Input: part model. Units: mm. Frame: model coordinates. A direction names the side the tool comes from. Coordinates: 2 decimals unless noted, no trailing zeros. Loops run counter-clockwise (first coordinate to the right, second up) from the corner with the lowest first, then second, coordinate; pieces in that order, holes last.
(1) Section C-C, the plane x = 3. Return loops of the section in (y, z), then the cut area to 3 significant figures.
(2) Contact query for flat-ended pins moving along their axis: P1, Ø3, axis at y = 16.5, z = 2, coming from the -X side; P2, Ø1.5, axis at y = -15, z = 4.5, coming from the -X side; P3, Ø1.1, axis at y = -20.5, z = 5.5, coming from the +X side. Output: stop coordinate, or through.
(3) Set-up query: faces 5 (the face through (-16.17, 16.26, 2.44)), 6 (the face through (-19.6, -10, 5.4)), 7 (the face through (10, -19.8, 5.4)), 8 (the face through (-10, 19.7, 5.4)), 9 (the face through (17.2, 12.4, 5.4)). Return all of +Z, -Z, +X, -X, +Y, -Y with unobstructed straight access to the full face (end or side cutting, diameter ignored); none if empty.
(4) Mould query, pull axis Y, two halves, no side actions, for faces 1 (the face through (17.2, -12.6, 5.4)), 2 (the face through (0, 0, 0.9)), 3 (the face through (-12.4, 16.86, 5.4)), 4 (the face through (12.6, -17.14, 5.4)). Classes: released by +Y, released by -Y, zero draft, split by the parting line, or undercut.
(5) Section B-B, the plane z = 3. Return loops of the section in (x, y).
(6) Section D-D, the plane x = -13.5. Return loops of the section in (y, z), then the cut area to 3 significant figures.
(7) Line query: L1, parallel to Y at x = 0, z = 4.4; L2, parallel to X at y = -0.5, z = 4.2. Output: solid intervals per line, ascending.
(8) Section A-A, the plane y = 0. Return loops of the section in (x, z).
Autodesk Inventor part; units mm, degrees
ref_plane "YZ Plane" through (0, 0, 0) normal (1, 0, 0) x (0, 1, 0)
ref_plane "XZ Plane" through (0, 0, 0) normal (0, 1, 0) x (-1, 0, 0)
ref_plane "XY Plane" through (0, 0, 0) normal (0, 0, 1) x (1, 0, 0)
ref_plane "Work Plane1" through (15.4052, 15.0652, 4.9) normal (0, 0, 1) x (0, 1, 0)
sketch "Sketch1" plane through (15.4052, 15.0652, 4.9) normal (0, 0, 1) x (0, 1, 0)
  circle A0 centre (5.7948, 15.4052) radius 2.5
  circle A1 centre (-15.6052, -5.7948) radius 2.5
  line L0 (-20.0856, 39.0762) -> (-20.0856, 40.2052)
  line L1 (-20.0856, 40.2052) -> (-38.2052, 40.2052)
  arc A2 (-38.2052, 40.2052) -> (-40.2052, 38.2052) centre (-38.2052, 38.2052) ccw
  line L2 (-40.2052, 20.2953) -> (-40.2052, 38.2052)
  line L3 (-40.2052, 20.2953) -> (-39.0783, 20.2953)
  arc A3 (-39.0783, 20.2953) -> (-38.6768, 20.6232) centre (-39.0783, 20.7051) ccw
  arc A4 (-34.5391, 20.2052) -> (-38.6768, 20.6232) centre (-36.6291, 20.2052) ccw
  line L4 (-34.5391, 20.2052) -> (-34.5391, 10.4067)
  arc A5 (-38.647, 9.8643) -> (-34.5391, 10.4067) centre (-36.6023, 10.2052) ccw
  line L5 (-38.647, 9.8643) -> (-38.6775, 9.9849)
  arc A6 (-38.6775, 9.9849) -> (-39.0762, 10.3249) centre (-39.083, 9.9131) ccw
  line L6 (-39.0762, 10.3249) -> (-40.2052, 10.3249)
  line L7 (-40.2052, -7.7948) -> (-40.2052, 10.3249)
  arc A7 (-40.2052, -7.7948) -> (-38.2052, -9.7948) centre (-38.2052, -7.7948) ccw
  line L8 (-38.2052, -9.7948) -> (-20.2052, -9.7948)
  line L9 (-20.2052, -9.7948) -> (-20.2052, -10.8453)
  arc A8 (-20.6052, -11.3352) -> (-20.2052, -10.8453) centre (-20.7052, -10.8453) ccw
  arc A9 (-20.6052, -11.3352) -> (-20.2052, -15.2948) centre (-20.2052, -13.2948) ccw
  line L10 (-20.2052, -15.2948) -> (-10.2052, -15.2948)
  arc A10 (-10.2052, -15.2948) -> (-9.8052, -11.3352) centre (-10.2052, -13.2948) ccw
  arc A11 (-10.2052, -10.8453) -> (-9.8052, -11.3352) centre (-9.7052, -10.8453) ccw
  line L11 (-10.2052, -10.8453) -> (-10.2052, -9.7948)
  line L12 (-10.2052, -9.7948) -> (7.7948, -9.7948)
  arc A12 (7.7948, -9.7948) -> (9.7948, -7.7948) centre (7.7948, -7.7948) ccw
  line L13 (9.7948, 10.2052) -> (9.7948, -7.7948)
  line L14 (9.7948, 10.2052) -> (10.8453, 10.2052)
  arc A13 (11.3352, 9.8052) -> (10.8453, 10.2052) centre (10.8453, 9.7052) ccw
  arc A14 (11.3352, 9.8052) -> (15.2948, 10.2052) centre (13.2948, 10.2052) ccw
  line L15 (15.2948, 10.2052) -> (15.2948, 20.2052)
  arc A15 (15.2948, 20.2052) -> (11.3352, 20.6052) centre (13.2948, 20.2052) ccw
  arc A16 (10.8453, 20.2052) -> (11.3352, 20.6052) centre (10.8453, 20.7052) ccw
  line L16 (10.8453, 20.2052) -> (9.7948, 20.2052)
  line L17 (9.7948, 38.2052) -> (9.7948, 20.2052)
  arc A17 (9.7948, 38.2052) -> (7.7948, 40.2052) centre (7.7948, 38.2052) ccw
  line L18 (7.7948, 40.2052) -> (-10.1151, 40.2052)
  line L19 (-10.1151, 40.2052) -> (-10.1151, 39.0783)
  arc A18 (-10.1151, 39.0783) -> (-9.7873, 38.6768) centre (-9.7054, 39.0783) ccw
  arc A19 (-10.2052, 34.5391) -> (-9.7873, 38.6768) centre (-10.2052, 36.6291) ccw
  line L20 (-10.2052, 34.5391) -> (-20.0038, 34.5391)
  arc A20 (-20.5462, 38.647) -> (-20.0038, 34.5391) centre (-20.2052, 36.6023) ccw
  line L21 (-20.5462, 38.647) -> (-20.4256, 38.6775)
  arc A21 (-20.4256, 38.6775) -> (-20.0856, 39.0762) centre (-20.4974, 39.083) ccw
  line L22 (-0.2052, 32.2052) -> (-30.2052, 32.2052)
  arc A22 (1.7948, 30.2052) -> (-0.2052, 32.2052) centre (-0.2052, 30.2052) ccw
  line L23 (1.7948, 30.2052) -> (1.7948, 0.2052)
  arc A23 (-0.2052, -1.7948) -> (1.7948, 0.2052) centre (-0.2052, 0.2052) ccw
  line L24 (-0.2052, -1.7948) -> (-30.2052, -1.7948)
  arc A24 (-32.2052, 0.2052) -> (-30.2052, -1.7948) centre (-30.2052, 0.2052) ccw
  line L25 (-32.2052, 0.2052) -> (-32.2052, 30.2052)
  arc A25 (-30.2052, 32.2052) -> (-32.2052, 30.2052) centre (-30.2052, 30.2052) ccw
  circle A26 centre (-35.2052, 35.2052) radius 2.425
  circle A27 centre (-29.7052, 36.0052) radius 2.65
  circle A28 centre (-36.0052, 29.7052) radius 2.65
  circle A29 centre (-35.2052, -4.7948) radius 2.425
  circle A30 centre (-29.7052, -5.5948) radius 2.65
  circle A31 centre (-36.0052, 0.7052) radius 2.65
  circle A32 centre (4.7948, 35.2052) radius 2.425
  circle A33 centre (-0.7052, 36.0052) radius 2.65
  circle A34 centre (5.5948, 29.7052) radius 2.65
  circle A35 centre (5.5948, 0.7052) radius 2.65
  circle A36 centre (-0.7052, -5.5948) radius 2.65
  circle A37 centre (4.7948, -4.7948) radius 2.425
  point P0 (-15.0652, 15.4052)
extrude "Extrusion1" add sketch "Sketch1" against normal blind 5 draft -1 contours A22 L23 A23 L24 A24 L25 A25 L22
sketch "Sketch2" plane through (15.4052, 15.0652, 4.9) normal (0, 0, 1) x (1, 0, 0)
  circle A0 centre (-26.2552, -7.0652) radius 3
  circle A1 centre (-26.2552, -23.0652) radius 3
  circle A2 centre (-4.2552, -15.0652) radius 1.6
  line L0 (-50.1952, -15.0652) -> (19.3848, -15.0652)
  circle A3 centre (-15.4052, -15.0652) radius 12
  dimension "d4" = 24
extrude "Extrusion2" cut sketch "Sketch2" against normal blind 4 contours A0 A3 | A0 A3 A2 L0 | A3 L0 A2 | L0 A2 A3 A1 | L0 A3 A2 | A1 A3 picked at (-24.6691, -8.292) picked at (-4.1694, -14.672) picked at (-4.1694, -15.4584) picked at (-24.6691, -21.8384)
sketch "Sketch4" plane through (15.4052, 15.0652, 4.9) normal (0, 0, 1) x (1, 0, 0)
  circle A0 centre (-15.4052, -15.0652) radius 12 construction
  line L0 (-32.2052, -0.2052) -> (-32.2052, -30.2052) construction
  arc A1 (-32.2052, -30.2052) -> (-30.2052, -32.2052) centre (-30.2052, -30.2052) ccw construction
  line L1 (-30.2052, -32.2052) -> (-0.2052, -32.2052) construction
  arc A2 (-0.2052, -32.2052) -> (1.7948, -30.2052) centre (-0.2052, -30.2052) ccw construction
  line L2 (1.7948, -30.2052) -> (1.7948, -0.2052) construction
  arc A3 (1.7948, -0.2052) -> (-0.2052, 1.7948) centre (-0.2052, -0.2052) ccw construction
  line L3 (-0.2052, 1.7948) -> (-30.2052, 1.7948) construction
  arc A4 (-30.2052, 1.7948) -> (-32.2052, -0.2052) centre (-30.2052, -0.2052) ccw construction
  line L4 (-37.9052, -25.0652) -> (7.0948, -25.0652) construction
  line L5 (7.0948, -25.0652) -> (7.0948, -5.0652) construction
  line L6 (7.0948, -5.0652) -> (-37.9052, -5.0652) construction
  line L7 (-37.9052, -5.0652) -> (-37.9052, -25.0652) construction
  line L8 (-37.9052, -25.0652) -> (7.0948, -5.0652) construction
  line L9 (7.0948, -25.0652) -> (-37.9052, -5.0652) construction
  line L10 (-25.4052, 7.4348) -> (-5.4052, 7.4348) construction
  line L11 (-5.4052, 7.4348) -> (-5.4052, -37.5652) construction
  line L12 (-5.4052, -37.5652) -> (-25.4052, -37.5652) construction
  line L13 (-25.4052, -37.5652) -> (-25.4052, 7.4348) construction
  line L14 (-25.4052, 7.4348) -> (-5.4052, -37.5652) construction
  line L15 (-5.4052, 7.4348) -> (-25.4052, -37.5652) construction
  line L16 (1.7075, -30.2052) -> (1.7075, -0.2052) construction
  line L17 (-30.2052, -32.2052) -> (-0.2052, -32.2052) construction
  line L18 (-32.118, -0.2052) -> (-32.118, -30.2052) construction
  line L19 (-0.2052, 1.7948) -> (-30.2052, 1.7948) construction
  line L20 (7.0948, -5.0652) -> (1.7075, -5.0652)
  line L21 (1.7075, -5.0652) -> (1.7075, -25.0652)
  line L22 (1.7075, -25.0652) -> (7.0948, -25.0652)
  line L23 (7.0948, -25.0652) -> (7.0948, -5.0652)
  line L24 (-5.4052, -37.5652) -> (-25.4052, -37.5652)
  line L25 (-25.4052, -37.5652) -> (-25.4052, -32.2052)
  line L26 (-25.4052, -32.2052) -> (-5.4052, -32.2052)
  line L27 (-5.4052, -32.2052) -> (-5.4052, -37.5652)
  line L28 (-32.2052, -25.0652) -> (-37.9052, -25.0652)
  line L29 (-37.9052, -25.0652) -> (-37.9052, -5.0652)
  line L30 (-37.9052, -5.0652) -> (-32.2052, -5.0652)
  line L31 (-32.2052, -5.0652) -> (-32.2052, -25.0652)
  line L32 (-25.4052, 1.7948) -> (-5.4052, 1.7948)
  line L33 (-5.4052, 1.7948) -> (-5.4052, 7.4348)
  line L34 (-5.4052, 7.4348) -> (-25.4052, 7.4348)
  line L35 (-25.4052, 7.4348) -> (-25.4052, 1.7948)
  point P0 (1.7948, -5.0652)
  point P1 (-5.4052, -32.2052)
  point P2 (-32.118, -5.0652)
  point P3 (-5.4052, 1.7948)
  dimension "d7" = 45
  dimension "d8" = 20
  dimension "d9" = 20
  dimension "d10" = 45
extrude "Extrusion4" add sketch "Sketch4" along normal blind 1
sketch "Sketch5" plane through (15.4052, 15.0652, 4.9) normal (0, 0, 1) x (1, 0, 0)
  line L0 (1.7075, -5.0652) -> (1.7948, -5.0652)
  line L1 (1.7948, -5.0652) -> (1.7948, -0.2052)
  arc A0 (1.7948, -0.2052) -> (-0.2052, 1.7948) centre (-0.2052, -0.2052) ccw
  line L2 (-0.2052, 1.7948) -> (-5.4052, 1.7948)
  line L3 (-5.4052, 1.7948) -> (-25.4052, 1.7948)
  line L4 (-25.4052, 1.7948) -> (-30.2052, 1.7948)
  arc A1 (-30.2052, 1.7948) -> (-32.2052, -0.2052) centre (-30.2052, -0.2052) ccw
  line L5 (-32.2052, -0.2052) -> (-32.2052, -5.0652)
  line L6 (-32.2052, -5.0652) -> (-32.2052, -25.0652)
  line L7 (-32.2052, -25.0652) -> (-32.2052, -30.2052)
  arc A2 (-32.2052, -30.2052) -> (-30.2052, -32.2052) centre (-30.2052, -30.2052) ccw
  line L8 (-30.2052, -32.2052) -> (-25.4052, -32.2052)
  line L9 (-25.4052, -32.2052) -> (-5.4052, -32.2052)
  line L10 (-5.4052, -32.2052) -> (-0.2052, -32.2052)
  arc A3 (-0.2052, -32.2052) -> (1.7948, -30.2052) centre (-0.2052, -30.2052) ccw
  line L11 (1.7948, -30.2052) -> (1.7948, -25.0652)
  line L12 (1.7948, -25.0652) -> (1.7075, -25.0652)
  line L13 (1.7075, -25.0652) -> (1.7075, -5.0652)
  circle A4 centre (-15.4052, -15.0652) radius 12
extrude "Extrusion5" add sketch "Sketch5" along normal blind 1
properties part number "30_Cube_counterplate_LEDmount"
Report:
1. outline: (-22.5, 4.9) - (-17.14, 4.9) - (-17.05, -0.1) - (16.77, -0.1) - (16.86, 4.9) - (22.5, 4.9) - (22.5, 5.9) - (11.62, 5.9) - (11.62, 0.9) - (-11.62, 0.9) - (-11.62, 5.9) - (-22.5, 5.9) - close
1. area: 98.4 mm2
2. P1: stops at x = -16.75
2. P2: stops at x = -16.8
2. P3: stops at x = 10
3. face 5: -Z, -X, +Y
3. face 6: +Z, -Z, -X, -Y
3. face 7: +Z, -Z, +X, -Y
3. face 8: +Z, -Z, -X, +Y
3. face 9: +Z, -Z, +X, +Y
4. face 1: zero draft
4. face 2: undercut
4. face 3: released by +Y
4. face 4: released by -Y
5. outline: (-16.77, -15.14) arc R1.97 ccw to (-14.8, -17.11) - (15.2, -17.11) arc R1.97 ccw to (17.17, -15.14) - (17.17, 14.86) arc R1.97 ccw to (15.2, 16.83) - (-14.8, 16.83) arc R1.97 ccw to (-16.77, 14.86) - close; hole circle Ø24 at (0, 0)
6. outline: (-17.14, 4.9) - (-17.05, -0.1) - (16.77, -0.1) - (16.86, 4.9) - (16.86, 5.9) - (-17.14, 5.9) - close
6. area: 204 mm2
7. L1: y = -17.13 to -12, 12 to 16.85
7. L2: x = -16.79 to -11.99, 11.99 to 17.19
8. outline: (-22.5, 4.9) - (-16.8, 4.9) - (-16.71, -0.1) - (17.11, -0.1) - (17.2, 4.9) - (22.5, 4.9) - (22.5, 5.9) - (12, 5.9) - (12, 0.9) - (-12, 0.9) - (-12, 5.9) - (-22.5, 5.9) - close
